from build123d import *

# Parameters (mm, degrees)
F0_W      = 1371.6
F0_H      = 1772.92
F1_DEPTH  = 1701.8
F2_W      = 736.6
F2_H      = 83.82
F3_DEPTH  = 1701.8
F4_W      = 267.8561401336
F4_H      = 1066.8
F5_DEPTH  = 762
F6_DEPTH  = 838.2
F7_R      = 80.01
F8_DEPTH  = 317.5
F10_DEPTH = 38.1
F11_DEPTH = 38.1


with BuildPart() as f1:
    # F0 (on Front) → F1 (new body)
    with BuildSketch(Plane.XZ):
        with Locations((638.0169455886, 557.9506990528)):
            Rectangle(F0_W, F0_H)
    extrude(amount=F1_DEPTH)

    # F2 (on face) → F3 (cut)
    with BuildSketch(Plane.XZ.offset(1701.8)):
        with Locations((955.5169455886, 1085.0006990528)):
            Rectangle(F2_W, F2_H)
        with BuildLine():
            Line((1323.8169455886, 115.9906990528), (1323.8169455886, 598.5906990528))
            Line((1323.8169455886, 598.5906990528), (1055.960805455, 598.5906990528))
            ThreePointArc((1055.960805455, 598.5906990528), (1104.1727493557, 482.1967702193), (1120.6169455886, 357.2906990528))
            ThreePointArc((1120.6169455886, 357.2906990528), (1104.1727493557, 232.3846278863), (1055.960805455, 115.9906990528))
            Line((1055.960805455, 115.9906990528), (1323.8169455886, 115.9906990528))
        make_face()
        with BuildLine():
            ThreePointArc((1120.6169455886, 357.2906990528), (1104.1727493557, 482.1967702193), (1055.960805455, 598.5906990528))
            ThreePointArc((1055.960805455, 598.5906990528), (220.0730857222, 598.5906990528), (638.0169455886, -125.3093009472))
            ThreePointArc((638.0169455886, -125.3093009472), (879.3169455886, -60.6531608136), (1055.960805455, 115.9906990528))
            ThreePointArc((1055.960805455, 115.9906990528), (1104.1727493557, 232.3846278863), (1120.6169455886, 357.2906990528))
        make_face()
    extrude(amount=-F3_DEPTH, mode=Mode.SUBTRACT)

    # F4 (on face) → F5 (cut)
    with BuildSketch(Plane.XY.offset(115.9906990528)):
        with Locations((1189.8888755218, -850.9)):
            Rectangle(F4_W, F4_H)
    extrude(amount=-F5_DEPTH, mode=Mode.SUBTRACT)

    # F6 (cut): a face of the model
    f6_faces = [f1.faces().sort_by_distance(p)[0] for p in [
        (1055.960805455, -850.9, -106.2593009472),
    ]]
    extrude(f6_faces, amount=-F6_DEPTH, mode=Mode.SUBTRACT)

    # F7 (on face) → F8 (cut)
    with BuildSketch(Plane.XY.offset(1444.4106990528)):
        with Locations((1112.9969455886, -850.9)):
            Circle(F7_R)
    extrude(amount=-F8_DEPTH, mode=Mode.SUBTRACT)

    # F9 (on face) → F10 (cut)
    with BuildSketch(Plane(origin=(-47.7830544114, 0, 0), x_dir=(0, -1, 0), z_dir=(-1, 0, 0))):
        Polygon((0, 1444.4106990528), (0, 1322.4906990528), (121.92, 1444.4106990528), align=None)
        Polygon((0, -206.5893009472), (0, -328.5093009472), (121.92, -328.5093009472), align=None)
        Polygon((1701.8, -206.5893009472), (1579.88, -328.5093009472), (1701.8, -328.5093009472), align=None)
        Polygon((1579.88, 1444.4106990528), (1701.8, 1322.4906990528), (1701.8, 1444.4106990528), align=None)
    extrude(amount=-F10_DEPTH, mode=Mode.SUBTRACT)

    # F9 (on face) → F11 (cut)
    with BuildSketch(Plane(origin=(-47.7830544114, 0, 0), x_dir=(0, -1, 0), z_dir=(-1, 0, 0))):
        Polygon((0, 1322.4906990528), (731.6059692308, 557.9506990528), (850.9, 682.6148791171), (121.92, 1444.4106990528), align=None)
        Polygon((731.6059692308, 557.9506990528), (850.9, 433.2865189885), (970.1940307692, 557.9506990528), (850.9, 682.6148791171), align=None)
        Polygon((850.9, 682.6148791171), (970.1940307692, 557.9506990528), (1701.8, 1322.4906990528), (1579.88, 1444.4106990528), align=None)
        Polygon((970.1940307692, 557.9506990528), (850.9, 433.2865189885), (1579.88, -328.5093009472), (1701.8, -206.5893009472), align=None)
        Polygon((0, -206.5893009472), (121.92, -328.5093009472), (850.9, 433.2865189885), (731.6059692308, 557.9506990528), align=None)
    extrude(amount=-F11_DEPTH, mode=Mode.SUBTRACT)


solid = f1.part
Geometry check sheet. Reference: the model listing, model coordinates, mm. A direction names the side the tool comes from. Give positions to 0.01 mm unless a question says otherwise; leave off trailing zeros. Write each loop counter-clockwise with the first axis right and the second up, starting at its lowest first coordinate (ties: lowest second). Pieces come first, ordered by that corner, then holes. Notation, with made-up numbers: M 2,2 L 7,2 A24 ccw 7,25 Z; hole C 55.25,27 d7. An arc over 180 degrees is marked long. Answer as CSV lines item,"result". Start each with the question number.
Q1. Release check for a two-part mould opening along X. For faces 1 (the face through (1149.92, -921.88, 1287.88)), 2 (the face through (-47.783, -841, 1143)), 3 (the face through (-29, -1210.29, 57.72)) record: pulls with the +X half, pulls with the -X half, needs draft (parallel to the pull), parting line crosses it, or undercut.
Q2. Material ranges on L1, parallel to Z at x = 1169.5, y = -734.5; L2, parallel to Z at x = 791.5, y = -161; L3, parallel to X at y = -850, z = 1245, recorded low to high.
Q3. Section check A-A, the plane x = 432. Record the cut outline in (y, z).
Q4. Section check B-B, the plane y = -891. Record the cut outline in (x, z), then the cut area to 3 significant figures.
Q5. Section check C-C, the plane z = -25. Record the cut outline in (x, y), then the cut area to 3 significant figures.
Q6. Go/stop test with flat-tipped pins: pin 1 (10 mm diameter, centred on x = 768, y = -1326, fed in from -Z); pin 2 (3 mm diameter, centred on x = 1052, y = -468.5, fed in from -Z); pin 3 (4 mm diameter, centred on y = -1193.5, z = -36, fed in from +X). Record where each tip stops, or that it passes through.
Q7. Tool access check on faces 4 (the face through (901, -1384.3, -153)), 5 (the face through (1188, -1545, 115.991)), 6 (the face through (324, 0, 767)), 7 (the face through (1323.817, -157, -109)), 8 (the face through (-29, -1331, 935)). Record the directions out of +Z, -Z, +X, -X, +Y, -Y that give a thin tool (end or side, any length) a straight path to the whole face; none if there is none.
Q8. Section check D-D, the plane x = 963. Record the cut outline in (y, z), then the cut area to 3 significant figures.
Geometry says:
1,face 1,"undercut"
1,face 2,"pulls with the -X half"
1,face 3,"needs draft"
2,L1,"598.59 to 1043.09, 1126.91 to 1444.41"
2,L2,"-328.51 to -100.25, 814.83 to 1043.09, 1126.91 to 1444.41"
2,L3,"-47.78 to 1032.99, 1193 to 1323.82"
3,outline,"M -1701.8,-328.51 L -1384.3,-328.51 L -1384.3,-79.13 L -1701.8,-79.13 Z; M -1701.8,793.71 L 0,793.71 L 0,1444.41 L -1701.8,1444.41 Z; M -317.5,-328.51 L 0,-328.51 L 0,-79.13 L -317.5,-79.13 Z"
4,outline,"M -47.78,-328.51 L 217.76,-328.51 L 217.76,115.99 L 220.07,115.99 A482.6 cw 1055.96,598.59 L 1323.82,598.59 L 1323.82,1043.09 L 587.22,1043.09 L 587.22,1126.91 L 1043.76,1126.91 L 1043.76,1444.41 L -47.78,1444.41 L -47.78,724.52 L -9.68,724.52 L -9.68,391.38 L -47.78,391.38 Z; M 1182.23,1126.91 L 1323.82,1126.91 L 1323.82,1444.41 L 1182.23,1444.41 Z"
4,area,"1,120,000 mm^2"
5,outline,"M -47.78,-1701.8 L 343.47,-1701.8 L 343.47,-1384.3 L 217.76,-1384.3 L 217.76,-317.5 L 343.47,-317.5 L 343.47,0 L -47.78,0 L -47.78,-173.77 L -9.68,-173.77 L -9.68,-412.36 L -47.78,-412.36 L -47.78,-1289.44 L -9.68,-1289.44 L -9.68,-1528.03 L -47.78,-1528.03 Z; M 932.56,-1701.8 L 1323.82,-1701.8 L 1323.82,-1384.3 L 932.56,-1384.3 Z; M 932.56,-317.5 L 1323.82,-317.5 L 1323.82,0 L 932.56,0 Z"
5,area,"762,000 mm^2"
6,pin 1,"z = 820.63"
6,pin 2,"z = 602.8"
6,pin 3,"x = 217.76"
7,face 4,"-Z, +X"
7,face 5,"+X, +Y, -Y"
7,face 6,"+Z, -Z, +X, -X, +Y"
7,face 7,"+Z, -Z, +X, +Y, -Y"
7,face 8,"-X"
8,outline,"M -1701.8,-328.51 L -1384.3,-328.51 L -1384.3,0.52 L -1701.8,0.52 Z; M -1701.8,714.07 L 0,714.07 L 0,1043.09 L -1701.8,1043.09 Z; M -1701.8,1126.91 L 0,1126.91 L 0,1444.41 L -1701.8,1444.41 Z; M -317.5,-328.51 L 0,-328.51 L 0,0.52 L -317.5,0.52 Z"
8,area,"1,310,000 mm^2"
